For this review, take the finished solid that the model builds, in its own axes (mm). A direction names the side the tool comes from. Coordinates: 2 decimals unless noted, no trailing zeros. Loops run counter-clockwise (first coordinate to the right, second up) from the corner with the lowest first, then second, coordinate; pieces in that order, holes last. Notation, with made-up numbers: M 64,19 L 71,19 A26 ccw 71,37 Z; hole C 2.25,2.25 d11. An arc over 180 degrees is marked long. Answer as a JSON object with one key per item and string values. Group by question number.
Item 1: Wall thickness on L1, parallel to X at y = -2.25, z = 1 (3 decimals); L2, parallel to Z at x = 44.5, y = -2.9; L3, parallel to X at y = -1.6, z = 110.5: over which ranges is each line inside the solid? List them lowest first. Write a range as from..to.
Item 2: Add section C-C (z = 51). State the section outline as (x, y) points (3 decimals), then the cut area to 3 significant figures.
Item 3: Tool access review of faces 4 (the face through (3, 0, 43)), 5 (the face through (15.875, -2, 39)): name each direction out of +Z, -Z, +X, -X, +Y, -Y from which nothing blocks a thin tool from reaching the whole face with its end or side.
Item 4: Add section B-B (x = 8). State the section outline as (y, z) points, then the cut area to 3 significant figures.
Item 5: Insertion check: pin 1 (5.5 mm diameter, centred on x = 0, z = 114.3, fed in from -Y); pin 2 (1 mm diameter, centred on x = 10.5, y = -2, fed in from -Z); pin 3 (7.5 mm diameter, centred on x = 0, z = 0, fed in from -Y); pin 4 (1.5 mm diameter, centred on y = -1, z = 29.5, fed in from +X) (3 decimals). Each pin has a flat end and moves straight along its axis. Give the tip position at first contact, or say it passes through.
Item 6: Add section A-A (y = -2.45). Count the separate pieces of the cut face and the enclosed holes in it, then the cut area to 3 significant figures.
Item 7: Mouldability with a two-part tool opening along X and no side actions: class faces 1 (the face through (-12.6, -1.5, 90.2)), 2 (the face through (18.27, -1.5, 10.2)), 3 (the face through (-3.863, -1.503, 96.787)) as +X half, -X half, draft (parallel to the pull), parting line (faces both ways), or undercut.
from build123d import *

# Parameters (mm, degrees)
F0_R     = 3.175
F1_DEPTH = 3.048


with BuildPart() as f1:
    # F0 (on Front) → F1 (new body)
    with BuildSketch(Plane.XZ):
        with BuildLine():
            ThreePointArc((3.175, 0), (-2.2450640303, -2.2450640303), (0, 3.175))
            Line((0, 3.175), (0, 9.525))
            ThreePointArc((0, 9.525), (-6.7351920908, 6.7351920908), (-9.525, 0))
            ThreePointArc((-9.525, 0), (-6.7351920908, -6.7351920908), (0, -9.525))
            Line((0, -9.525), (0.6773435479, -9.500885786))
            ThreePointArc((0.6773435479, -9.500885786), (6.9705567315, -6.4912990883), (9.525, 0))
            Line((9.525, 0), (3.175, 0))
        make_face()
        with BuildLine():
            ThreePointArc((-9.525, 0), (-6.7351920908, 6.7351920908), (0, 9.525))
            Line((0, 9.525), (0, 47.625))
            ThreePointArc((0, 47.625), (-10.0526499203, 51.2134278751), (-15.5606435644, 60.3564356436))
            Line((-15.5606435644, 60.3564356436), (-9.525, 0))
        make_face()
        with BuildLine():
            Line((0, 47.625), (0, 9.525))
            ThreePointArc((0, 9.525), (6.7351920908, 6.7351920908), (9.525, 0))
            Line((9.525, 0), (36.5125, 0))
            ThreePointArc((36.5125, 0), (38.8373399243, 5.6126600757), (44.45, 7.9375))
            Line((44.45, 7.9375), (23.8252, 7.9375))
            ThreePointArc((23.8252, 7.9375), (18.2035596682, 10.2660596682), (15.875, 15.8877))
            Line((15.875, 15.8877), (15.875, 63.5))
            ThreePointArc((15.875, 63.5), (11.2253201513, 52.2746798487), (0, 47.625))
        make_face()
        with BuildLine():
            Line((36.5125, 0), (9.525, 0))
            ThreePointArc((9.525, 0), (6.9705567315, -6.4912990883), (0.6773435479, -9.500885786))
            Line((0.6773435479, -9.500885786), (44.7324052746, -7.9324746146))
            ThreePointArc((44.7324052746, -7.9324746146), (38.9380895153, -5.7116327839), (36.5125, 0))
        make_face()
        with BuildLine():
            ThreePointArc((-15.5606435644, 60.3564356436), (-10.0526499203, 51.2134278751), (0, 47.625))
            Line((0, 47.625), (0, 60.325))
            ThreePointArc((0, 60.325), (-3.175, 63.5), (0, 66.675))
            Line((0, 66.675), (0, 79.375))
            ThreePointArc((0, 79.375), (-10.4912828548, 75.4142187767), (-15.7474569047, 65.5082893304))
            ThreePointArc((-15.7474569047, 65.5082893304), (-15.8430821396, 64.5061676396), (-15.875, 63.5))
            Line((-15.875, 63.5), (-15.5606435644, 60.3564356436))
        make_face()
        with BuildLine():
            Line((0, 60.325), (0, 47.625))
            ThreePointArc((0, 47.625), (11.2253201513, 52.2746798487), (15.875, 63.5))
            ThreePointArc((15.875, 63.5), (15.8430821396, 64.5061676396), (15.7474569047, 65.5082893304))
            ThreePointArc((15.7474569047, 65.5082893304), (10.4912828548, 75.4142187767), (0, 79.375))
            Line((0, 79.375), (0, 66.675))
            ThreePointArc((0, 66.675), (2.2450640303, 65.7450640303), (3.175, 63.5))
            ThreePointArc((3.175, 63.5), (2.2450640303, 61.2549359697), (0, 60.325))
        make_face()
        with BuildLine():
            ThreePointArc((44.45, 7.9375), (38.8373399243, 5.6126600757), (36.5125, 0))
            ThreePointArc((36.5125, 0), (38.9380895153, -5.7116327839), (44.7324052746, -7.9324746146))
            ThreePointArc((44.7324052746, -7.9324746146), (50.1616327839, -5.5119104847), (52.3875, 0))
            ThreePointArc((52.3875, 0), (50.0626600757, 5.6126600757), (44.45, 7.9375))
        make_face()
        with BuildLine():
            ThreePointArc((47.625, 0), (44.45, -3.175), (41.275, 0))
            ThreePointArc((41.275, 0), (44.45, 3.175), (47.625, 0))
        make_face(mode=Mode.SUBTRACT)
        with BuildLine():
            ThreePointArc((0, -9.525), (0.3388863295, -9.5189695375), (0.6773435479, -9.500885786))
            Line((0.6773435479, -9.500885786), (0, -9.525))
        make_face()
        with BuildLine():
            ThreePointArc((-15.875, 63.5), (-15.7962153946, 61.9203784605), (-15.5606435644, 60.3564356436))
            Line((-15.5606435644, 60.3564356436), (-15.875, 63.5))
        make_face()
        with BuildLine():
            ThreePointArc((0, 79.375), (10.4912828548, 75.4142187767), (15.7474569047, 65.5082893304))
            Line((15.7474569047, 65.5082893304), (9.525, 114.3))
            ThreePointArc((9.525, 114.3), (6.7351920908, 107.5648079092), (0, 104.775))
            Line((0, 104.775), (0, 99.886942851))
            Line((0, 99.886942851), (0, 79.375))
        make_face()
        with BuildLine():
            ThreePointArc((-15.7474569047, 65.5082893304), (-10.4912828548, 75.4142187767), (0, 79.375))
            Line((0, 79.375), (0, 99.886942851))
            Line((0, 99.886942851), (0, 104.775))
            ThreePointArc((0, 104.775), (-6.7351920908, 107.5648079092), (-9.525, 114.3))
            Line((-9.525, 114.3), (-15.7474569047, 65.5082893304))
        make_face()
        with Locations((-3.175, 99.886942851)):
            Circle(F0_R, mode=Mode.SUBTRACT)
        with BuildLine():
            ThreePointArc((0, 104.775), (6.7351920908, 107.5648079092), (9.525, 114.3))
            ThreePointArc((9.525, 114.3), (0, 123.825), (-9.525, 114.3))
            ThreePointArc((-9.525, 114.3), (-6.7351920908, 107.5648079092), (0, 104.775))
        make_face()
        with BuildLine():
            ThreePointArc((3.175, 114.3), (2.2450640303, 112.0549359697), (0, 111.125))
            ThreePointArc((0, 111.125), (-2.2450640303, 116.5450640303), (3.175, 114.3))
        make_face(mode=Mode.SUBTRACT)
        with BuildLine():
            Line((0, 9.525), (0, 3.175))
            ThreePointArc((0, 3.175), (2.2450640303, 2.2450640303), (3.175, 0))
            Line((3.175, 0), (9.525, 0))
            ThreePointArc((9.525, 0), (6.7351920908, 6.7351920908), (0, 9.525))
        make_face()
    extrude(amount=F1_DEPTH)


solid = f1.part
From the geometry:
{
 "1": {"L1": "x = -9.625..-3.013, 3.013..41.437, 47.463..52.324", "L2": "z = -7.94..-3.17, 3.17..7.94", "L3": "x = -10.01..10.01"},
 "2": {"outline": "M -14.625,-3.048 L 15.875,-3.048 L 15.875,0 L -14.625,0 Z", "area": "93.0 mm²"},
 "3": {"face 4": "+Z, -Z, +X, -X, +Y", "face 5": "+Z, +X, +Y, -Y"},
 "4": {"outline": "M -3.05,-9.24 L 0,-9.24 L 0,119.47 L -3.05,119.47 Z", "area": "392 mm²"},
 "5": {"pin 1": "passes through", "pin 2": "stops at z = -9.17", "pin 3": "stops at y = -3.05", "pin 4": "stops at x = 15.875"},
 "6": {"separate pieces": "1", "enclosed holes": "5", "area": "3,890 mm²"},
 "7": {"face 1": "-X half", "face 2": "+X half", "face 3": "undercut"}
}
